Build history of the part. All positions in model axes, mm. Coordinates: 2 decimals unless noted, no trailing zeros. Loops run counter-clockwise (first coordinate to the right, second up) from the corner with the lowest first, then second, coordinate; pieces in that order, holes last. Notation, with made-up numbers: (-12.75, 82.25) - (41.25, 82.25) arc R27 ccw to (41.25, 120.25) - close; hole circle Ø2 at (82.25, 47.5). An arc over 180 degrees is marked (long way). One line per item, written item: value.
```python
from build123d import *

# Parameters (mm, degrees)
F0_W     = 101.6
F0_H     = 101.6
F1_DEPTH = 25.4
F2_R     = 23.7572647181
F3_DEPTH = 25.401
F4_R     = 5.08
F5_R     = 5.08
F6_SIZE  = 12.7


with BuildPart() as f1:
    # F0 (on Top) → F1 (new body)
    with BuildSketch(Plane.XY):
        Rectangle(F0_W, F0_H)
    extrude(amount=-F1_DEPTH)

    # F2 (on face) → F3 (cut, through all)
    with BuildSketch(Plane.XY):
        Circle(F2_R)
    extrude(amount=-F3_DEPTH, mode=Mode.SUBTRACT)

    # F4
    f4_edges = [f1.edges().sort_by_distance(p)[0] for p in [
        (50.8, -50.8, -12.7),
        (-50.8, -50.8, -12.7),
        (50.8, 50.8, -12.7),
        (-23.757265, 0, 0),
        (-50.8, 50.8, -12.7),
    ]]
    fillet(f4_edges, radius=F4_R)

    # F5
    f5_edges = [f1.edges().sort_by_distance(p)[0] for p in [
        (-50.8, 0, 0),
        (-50.8, 45.72, -12.7),
        (-50.8, -45.72, -12.7),
        (-50.8, 0, -25.4),
    ]]
    fillet(f5_edges, radius=F5_R)

    # F6
    f6_edges = [f1.edges().sort_by_distance(p)[0] for p in [
        (-23.757265, 0, -25.4),
        (-23.757265, 0, -5.08),
    ]]
    chamfer(f6_edges, length=F6_SIZE)


solid = f1.part
```
Item 1: Pull direction X, two halves, no side cores. Call faces 1 (the face through (23.25, 7.32, -13.32)), 2 (the face through (49.272, -49.351, -12.807)), 3 (the face through (-49.351, 0.64, -1.528)): released by +X, released by -X, zero draft, split by the parting line, or undercut.
Check result:
face 1: undercut
face 2: released by +X
face 3: released by -X
Item 2: Probe probe 1 along Y at (x, z) = (0, -9); probe 2 along X at (y, z) = (-9.5, -10.5); probe 3 along Y at (x, z) = (-3.5, -9). List the from-to ranges inside material, lowest first. Write a range as from..to.
Check result:
probe 1: y = -50.8..-23.76, 23.76..50.8
probe 2: x = -50.8..-21.78, 21.78..50.8
probe 3: y = -50.8..-23.5, 23.5..50.8
Item 3: Drop flat-ended pins along their axis: P1, Ø2, axis at y = 33, z = -4.5, coming from the -X side; P2, Ø2, axis at y = 11, z = -21.5, coming from the +X side. Give the stop position or say it passes through.
Check result:
P1: stops at x = -50.8
P2: stops at x = 50.8
Item 4: Cut at A-A, the plane y = 0. Write the cut outline in (x, z).
Check result:
outline: (-50.8, -20.32) arc R5.08 ccw to (-45.72, -25.4) - (-36.46, -25.4) - (-23.76, -12.7) - (-23.76, -5.08) arc R5.08 ccw to (-28.84, 0) - (-45.72, 0) arc R5.08 ccw to (-50.8, -5.08) - close; (23.76, -12.7) - (36.46, -25.4) - (45.72, -25.4) arc R5.08 ccw to (50.8, -20.32) - (50.8, -5.08) arc R5.08 ccw to (45.72, 0) - (28.84, 0) arc R5.08 ccw to (23.76, -5.08) - close
